Can you work these out from the model? Positions are in its coordinate system, mm. Face numbers are marked on the shaded views. A direction names the side the tool comes from. Round coordinates to 2 decimals unless told otherwise and drop trailing zeros. Order: outer loops, then holes, each group sorted by start corner. A loop starts at its lowest first (then second) coordinate and runs counter-clockwise, first axis right, second up. Notation, with made-up numbers: M 19.5,-26.75 L 33.5,-26.75 A24 ccw 33.5,-4.75 Z; hole C 37.5,57.5 d5. An arc over 180 degrees is marked long. One line per question, with ' | ' between items.
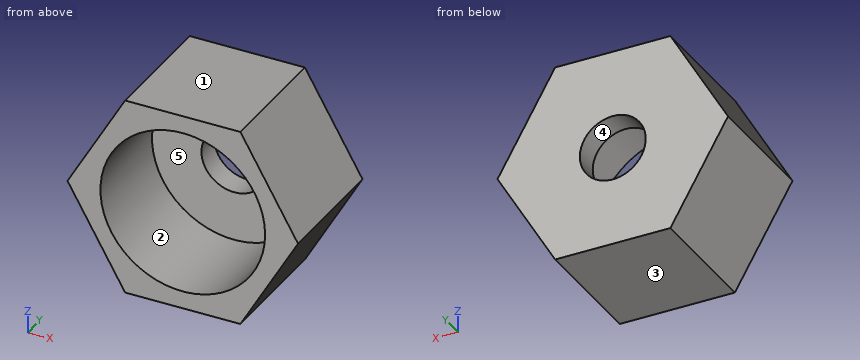
```python
from build123d import *

# Parameters (mm, degrees)
BOSS_EXTRUDE1_DEPTH = 7.5
SKETCH2_R           = 10
CUT_EXTRUDE2_DEPTH  = 12
SKETCH3_R           = 4
CUT_EXTRUDE3_DEPTH  = 16


with BuildPart() as part:
    # Sketch1 → Boss-Extrude1 (new body, symmetric)
    with BuildSketch(Plane(origin=(0, 0, 0), x_dir=(1, 0, 0), z_dir=(0, 1, 0))):
        Polygon((-14, 0), (-7, -12.124355653), (7, -12.124355653), (14, 0), (7, 12.124355653), (-7, 12.124355653), align=None)
    extrude(amount=BOSS_EXTRUDE1_DEPTH, both=True)

    # Sketch2 → Cut-Extrude2 (cut)
    with BuildSketch(Plane.XZ.offset(7.5)):
        Circle(SKETCH2_R)
    extrude(amount=-CUT_EXTRUDE2_DEPTH, mode=Mode.SUBTRACT)

    # Sketch3 → Cut-Extrude3 (cut, through all)
    with BuildSketch(Plane(origin=(0, 7.5, 0), x_dir=(1, 0, 0), z_dir=(0, 1, 0))):
        Circle(SKETCH3_R)
    extrude(amount=-CUT_EXTRUDE3_DEPTH, mode=Mode.SUBTRACT)


solid = part.part
```
(1) If we section it at D-D on z = 5.5: Please give me the cut outline in (x, y).
Final values:
outline: M -10.82,-7.5 L -8.35,-7.5 L -8.35,4.5 L 8.35,4.5 L 8.35,-7.5 L 10.82,-7.5 L 10.82,7.5 L -10.82,7.5 Z
(2) Please list where these lines run through material, in increasing order: probe 1 along Z at (x, y) = (0, -3.25); probe 2 along Y at (x, z) = (-8, 4); probe 3 along Z at (x, y) = (0, 6.7). Write a range as [from, to].
Final values:
probe 1: [-12.12, -10], [10, 12.12] | probe 2: [4.5, 7.5] | probe 3: [-12.12, -4], [4, 12.12]
(3) Thinking about a two-plate mould opening in Z: for the marked faces 1, 2 and 3, which applies, released by +Z, released by -Z, zero draft, split by the parting line, or undercut?
Final values:
face 1: released by +Z | face 2: undercut | face 3: released by -Z
(4) Will these pins go through, and if not, where does the flat tip stop? pin 1 Ø3 at (x, z) = (2, -7) entering from -Y; pin 2 Ø6 at (x, y) = (11, -4) entering from -Z.
Final values:
pin 1: y = 4.5 | pin 2: z = -10.39
(5) If we section it at C-C on z = 1.5: Please give me the cut outline in (x, y).
Final values:
outline: M -13.13,-7.5 L -9.89,-7.5 L -9.89,4.5 L -3.71,4.5 L -3.71,7.5 L -13.13,7.5 Z; M 3.71,4.5 L 9.89,4.5 L 9.89,-7.5 L 13.13,-7.5 L 13.13,7.5 L 3.71,7.5 Z
(6) On a 3-axis mill with a long thin cutter (end or side, diameter ignored), from which of +Z, -Z, +X, -X, +Y, -Y can I reach the whole of each face in a straight line? I mean the marked faces 4 and 5. Say none if no direction works.
Final values:
face 4: +Y, -Y | face 5: -Y
(7) If we section it at B-B on x = 0: Please give me the cut outline in (y, z).
Final values:
outline: M -7.5,-12.12 L 7.5,-12.12 L 7.5,-4 L 4.5,-4 L 4.5,-10 L -7.5,-10 Z; M -7.5,10 L 4.5,10 L 4.5,4 L 7.5,4 L 7.5,12.12 L -7.5,12.12 Z
(8) If we section it at A-A on y = -4.75: Please give me the cut outline in (x, z).
Final values:
outline: M -14,0 L -7,-12.12 L 7,-12.12 L 14,0 L 7,12.12 L -7,12.12 Z; hole C 0,0 d20
